from build123d import *

# Parameters (mm, degrees)
SKETCH1_R               = 6
BOSS_EXTRUDE1_DEPTH     = 10
SKETCH2_R               = 4
CUT_EXTRUDE1_DEPTH      = 14.114877049
CUT_EXTRUDE4_DEPTH      = 14.114877049
CUT_EXTRUDE4_DEPTH_BACK = 14.114877049
SKETCH3_W               = 2
SKETCH3_H               = 2


with BuildPart() as part:
    # Sketch1 → Boss-Extrude1 (new body)
    with BuildSketch(Plane.XY):
        Circle(SKETCH1_R)
    extrude(amount=BOSS_EXTRUDE1_DEPTH)

    # Sketch2 → Cut-Extrude1 (cut, through all)
    with BuildSketch(Plane.XY.offset(10)):
        Circle(SKETCH2_R)
    extrude(amount=-CUT_EXTRUDE1_DEPTH, mode=Mode.SUBTRACT)

    # Sketch3 → Cut-Extrude4 (cut, two sides: drawn at the far end of the back side and taken through both)
    with BuildSketch(Plane(origin=(0, 0, 0), x_dir=(1, 0, 0), z_dir=(0, 1, 0)).offset(-CUT_EXTRUDE4_DEPTH_BACK)):
        with Locations((0, -9)):
            Rectangle(SKETCH3_W, SKETCH3_H)
    extrude(amount=CUT_EXTRUDE4_DEPTH + CUT_EXTRUDE4_DEPTH_BACK, mode=Mode.SUBTRACT)


solid = part.part
Verification items for the finished model (mm, model axes). A direction names the side the tool comes from. Round coordinates to 2 decimals unless told otherwise and drop trailing zeros. Write each loop counter-clockwise with the first axis right and the second up, starting at its lowest first coordinate (ties: lowest second). Pieces come first, ordered by that corner, then holes.
(1) Section check C-C (z = 1). Enter the section's corners in (x, y).
Returned:
outline: circle Ø12 at (0, 0); hole circle Ø8 at (0, 0)
(2) Section check D-D (y = 5.75). Enter the section's corners in (x, z), plus the area to 3 significant figures.
Returned:
outline: (-1.71, 0) - (1.71, 0) - (1.71, 10) - (1, 10) - (1, 8) - (-1, 8) - (-1, 10) - (-1.71, 10) - close
area: 30.3 mm2
(3) Section check B-B (y = -1). Enter the section's corners in (x, z).
Returned:
outline: (-5.92, 0) - (-3.87, 0) - (-3.87, 10) - (-5.92, 10) - close; (3.87, 0) - (5.92, 0) - (5.92, 10) - (3.87, 10) - close
(4) Access from +Z, -Z, +X, -X, +Y, -Y to the whole of each face (thin tool, end or side, straight path). Record for faces 1 (the flat face through (0, -5, 8)), 2 (the flat face through (-1.42, -3.92, 0)).
Returned:
face 1: +Z, +Y, -Y
face 2: -Z, +X, -X, +Y, -Y
(5) Depth check by flat-ended pin: pin 1 Ø5 at (x, y) = (0, 0) entering from +Z; pin 2 Ø1 at (y, z) = (-5, 9) entering from -X; pin 3 Ø0.6 at (x, y) = (0, -5.5) entering from +Z; pin 4 Ø2 at (y, z) = (-2, 6.5) entering from -X. Enter the tip coordinate at first touch or a pass-through.
Returned:
pin 1: passes through
pin 2: stops at x = -3.97
pin 3: stops at z = 8
pin 4: stops at x = -5.92
(6) Section check A-A (x = 0). Enter the section's corners in (y, z).
Returned:
outline: (-6, 0) - (-4, 0) - (-4, 8) - (-6, 8) - close; (4, 0) - (6, 0) - (6, 8) - (4, 8) - close
(7) Mould release check, pull along Y, two halves, no side actions. Record for faces 3 (the flat face through (-1, -5, 9)), 4 (the cylindrical face through (-1.301, -5.857, 4.93)), 5 (the cylindrical face through (3.695, -1.532, 5.07)): pulls with the +Y half, pulls with the -Y half, needs draft (parallel to the pull), parting line crosses it, or undercut.
Returned:
face 3: needs draft
face 4: parting line crosses it
face 5: undercut
(8) Material ranges on line 1 (Y direction, x = 0, z = 4.5); line 2 (X direction, y = 1, z = 5); line 3 (X direction, y = 3, z = 7.75), recorded low to high.
Returned:
line 1: y = -6 to -4, 4 to 6
line 2: x = -5.92 to -3.87, 3.87 to 5.92
line 3: x = -5.2 to -2.65, 2.65 to 5.2
